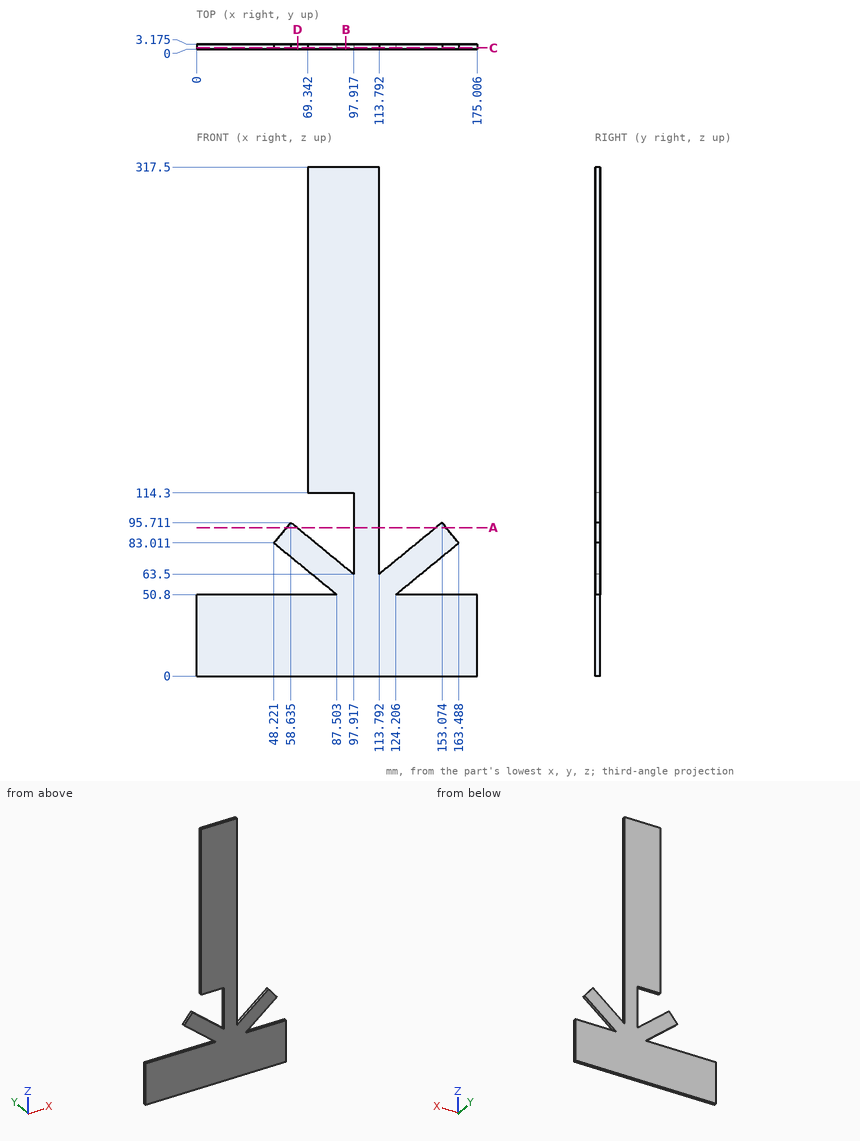
Study the drawing (mm; zero at the part's minimum x, y, z) and answer. Give positions to 0.01 mm unless a question says otherwise; leave off trailing zeros. Order: outer loops, then holes, each group sorted by start corner. A loop starts at its lowest first (then second) coordinate and runs counter-clockwise, first axis right, second up. Notation, with made-up numbers: (72, 55) - (122, 55) arc R32 cw to (122, 89) - close; hole circle Ø2 at (28.25, 89.5). An arc over 180 degrees is marked (long way). Answer in a Markdown table with one row per item. Add a question column.
Q1. The part is cut by section D-D (x = 63). Determine the outline of the cut face in (y, z) (1 decimal), then the cut area to 3 significant figures.
Q2. The part is cut by section B-B (x = 93). Determine the outline of the cut face in (y, z) (1 decimal).
Q3. Find the intervals of material crossed by line 1 along X through (y, z) = (1.75, 70); line 2 along Z through (x, y) = (20.5, 2.25); line 3 along X through (y, z) = (0.25, 253), in increasing order. Write a range as [from, to].
Q4. The part is cut by section A-A (z = 92.5). Determine the outline of the cut face in (x, y) (1 decimal).
Q5. The part is cut by section C-C (y = 0.75). Determine the outline of the cut face in (x, z) (1 decimal), then the cut area to 3 significant figures.
Q6. Given P1, Ø1.6, axis at y = 1, z = 83.5, coming from the -X side; P2, Ø1, axis at y = 1.5, z = 235.5, coming from the -X side; P3, Ø1, axis at x = 145, y = 2, coming from the +Z side, each flat-ended and moving along its own axis, determine where each tip first touches the part or whether it passes through.
Determined:
| question | item | result |
|---|---|---|
| 1 | outline | (0, 0) - (3.2, 0) - (3.2, 50.8) - (0, 50.8) - close; (0, 70.9) - (3.2, 70.9) - (3.2, 92.1) - (0, 92.1) - close |
| 1 | area | 229 mm² |
| 2 | outline | (0, 0) - (3.2, 0) - (3.2, 67.5) - (0, 67.5) - close; (0, 114.3) - (3.2, 114.3) - (3.2, 317.5) - (0, 317.5) - close |
| 3 | line 1 | x = [64.09, 89.99], [97.92, 113.79], [121.72, 147.62] |
| 3 | line 2 | z = [0, 50.8] |
| 3 | line 3 | x = [69.34, 113.79] |
| 4 | outline | (56, 0) - (62.6, 0) - (62.6, 3.2) - (56, 3.2) - close; (97.9, 0) - (113.8, 0) - (113.8, 3.2) - (97.9, 3.2) - close; (149.2, 0) - (155.7, 0) - (155.7, 3.2) - (149.2, 3.2) - close |
| 5 | outline | (0, 0) - (175, 0) - (175, 50.8) - (124.2, 50.8) - (163.5, 83) - (153.1, 95.7) - (113.8, 63.5) - (113.8, 317.5) - (69.3, 317.5) - (69.3, 114.3) - (97.9, 114.3) - (97.9, 63.5) - (58.6, 95.7) - (48.2, 83) - (87.5, 50.8) - (0, 50.8) - close |
| 5 | area | 20,700 mm² |
| 6 | P1 | stops at x = 48.22 |
| 6 | P2 | stops at x = 69.34 |
| 6 | P3 | stops at z = 89.5 |
